The model under review builds one solid part; all positions refer to its coordinate system, in mm. A direction names the side the tool comes from. Give positions to 0.01 mm unless a question says otherwise; leave off trailing zeros. Order: outer loops, then holes, each group sorted by start corner. A loop starts at its lowest first (then second) coordinate and runs counter-clockwise, first axis right, second up. Notation, with made-up numbers: (31, 42) - (66, 42) arc R18 ccw to (66, 49) - close; hole circle Ø2 at (7, 36.25). An arc over 180 degrees is marked (long way). Use CSV: the item, a comma, the result in double quotes.
Autodesk Inventor part; units mm, degrees
ref_plane "YZ Plane" through (0, 0, 0) normal (1, 0, 0) x (0, 1, 0)
ref_plane "XZ Plane" through (0, 0, 0) normal (0, 1, 0) x (-1, 0, 0)
ref_plane "XY Plane" through (0, 0, 0) normal (0, 0, 1) x (1, 0, 0)
sketch "Schizzo1" plane through (0, 0, 0) normal (0, 0, 1) x (1, 0, 0)
  line L0 (-42.5, 0) -> (42.5, 0)
  line L1 (-42.5, 0) -> (-42.5, 4)
  line L2 (-42.5, 4) -> (-32.5, 4)
  line L3 (-32.5, 4) -> (-32.5, 10)
  line L4 (-32.5, 10) -> (32.5, 10)
  line L5 (32.5, 10) -> (32.5, 4)
  line L6 (32.5, 4) -> (42.5, 4)
  line L7 (42.5, 4) -> (42.5, 0)
  point P0 (0, 0)
  point P1 (0, 0)
  point P2 (0, 10)
  dimension "d0" = 8
  dimension "d1" = 10
  dimension "d2" = 20
  dimension "d3" = 65
  dimension "d4" = 10
revolve "Rivoluzione1" add sketch "Schizzo1" angle 360 about axis through (-42.5, 0, 0) along (1, 0, 0)
chamfer "Smusso1" distance 0.5 angle 45 2 edges at (-42.5, -4, 0) (42.5, -4, 0)
thread "Filettatura1"
chamfer "Smusso2" distance 1 angle 45 2 edges at (-32.5, -10, 0) (32.5, -10, 0)
properties part number "Albero cuscinetto"
Item 1: Clearance check with flat-ended pins moving along their axes: pin 1 (1.5 mm diameter, centred on x = 16, y = -2.5, fed in from +Z); pin 2 (6 mm diameter, centred on x = 8, y = -5.5, fed in from -Z); pin 3 (5 mm diameter, centred on x = -0.5, z = -5.5, fed in from +Y). State where each tip first meets the part, or that it passes through.
Results list:
pin 1,"stops at z = 9.85"
pin 2,"stops at z = -9.68"
pin 3,"stops at y = 9.54"
Item 2: Take a section at C-C, the plane x = 0.5. Give the boundary of the cut face in (y, z).
Results list:
outline,"circle Ø20 at (0, 0)"
Item 3: Tool access review of faces 1 (the face through (32.5, 2, -4)), 2 (the face through (-42.5, 0, 0)), 3 (the face through (-32.5, 2, -4)): name each direction out of +Z, -Z, +X, -X, +Y, -Y from which nothing blocks a thin tool from reaching the whole face with its end or side.
Results list:
face 1,"+X"
face 2,"+Z, -Z, -X, +Y, -Y"
face 3,"-X"
Item 4: Take a section at A-A, the plane y = 0. Give the boundary of the cut face in (x, z), and give its area (3 significant figures).
Results list:
outline,"(-42.5, -3.5) - (-42, -4) - (-32.5, -4) - (-32.5, -9) - (-31.5, -10) - (31.5, -10) - (32.5, -9) - (32.5, -4) - (42, -4) - (42.5, -3.5) - (42.5, 3.5) - (42, 4) - (32.5, 4) - (32.5, 9) - (31.5, 10) - (-31.5, 10) - (-32.5, 9) - (-32.5, 4) - (-42, 4) - (-42.5, 3.5) - close"
area,"1,460 mm2"
Item 5: Wall thickness on L1, parallel to X at y = -6.25, z = -1; L2, parallel to Z at x = -0.5, y = -0.25: over which ranges is each line inside the solid? List them lowest first.
Results list:
L1,"x = -32.5 to 32.5"
L2,"z = -10 to 10"
